Source: CAD feature listing. Evaluate the final solid. Frame: model axes, mm. A direction names the side the tool comes from. Give positions to 0.01 mm unless a question says otherwise; leave off trailing zeros. Write each loop counter-clockwise with the first axis right and the second up, starting at its lowest first coordinate (ties: lowest second). Pieces come first, ordered by that corner, then holes. Notation, with made-up numbers: (-2, 20) -> (30, 20) arc R6 cw to (30, 31) -> close; hole circle Ø11 at (69.5, 66.25). An arc over 180 degrees is marked (long way). Use one line per item in the form item = value. Start each with the question number.
(1) Cut plane B-B, the plane z = -13. Count the separate pieces of the cut face and the enclosed holes in it, and give its area (3 significant figures).
(2) Material intervals for line 1 along Y through (x, z) = (0, 4); line 2 along X through (y, z) = (0, -3); line 3 along Y through (x, z) = (133, -11), sorted ascending. Write a range as from..to.
(3) Set-up query: faces 1 (the face through (100.9, 55.1, 0.3)), 2 (the face through (35.22, 1.93, 0.28)), 3 (the face through (131.72, 80.96, 0.28)). Return all of +Z, -Z, +X, -X, +Y, -Y with unobstructed straight access to the full face (end or side cutting, diameter ignored); none if empty.
(4) First-contact query: P1, Ø1.5, axis at x = 85.5, z = -0.5, coming from the +Y side; P2, Ø12, axis at x = 58, z = -8, coming from the -Y side; P3, Ø4, axis at x = 93, z = -11, coming from the -Y side. Flat tips, straight axial feed; report the tip coordinate or a pass-through.
(5) Draft query along X for faces 4 (the face through (-4.515, -3.462, 0.284)), 5 (the face through (19.249, 26.736, 0.284)), 6 (the face through (125, 83, -20.32)). Return one class per face: pulls with the +X half, pulls with the -X half, needs draft (parallel to the pull), parting line crosses it, or undercut.
(6) Cut plane A-A, the plane x = 0. Output: boundary loops of the cut face in (y, z), and give its area (3 significant figures).
from build123d import *

# Parameters (mm, degrees)
SKETCH1_R                       = 10.16
BOSS_EXTRUDE1_DEPTH             = 20.32
BOSS_EXTRUDE1_DEPTH_BACK        = 20.32
CUT_EXTRUDE2_DEPTH              = 85.09
CUT_EXTRUDE2_DEPTH_BACK         = 85.09
BOSS_EXTRUDE2_REACH             = 22.32
SKETCH4_R                       = 10.16
SKETCH4_R_2                     = 5.690130056
BOSS_EXTRUDE2_DIRECTION_2_REACH = 22.32


with BuildPart() as part:
    # Sketch1 → Boss-Extrude1 (new body, two sides)
    with BuildSketch(Plane.XY) as boss_extrude1_sk:
        with BuildLine():
            Line((-6.540792976, 16.533191684), (60.990787353, 43.249756441))
            Line((60.990787353, 43.249756441), (111.219656073, 79.494763154))
            add(Edge.make_bspline(
                [(111.219656073, 79.494763154), (115.143809103, 89.538582986), (111.485189552, 100.079798905)],
                knots=[0, 0, 0, 1, 1, 1], degree=2))
            add(Edge.make_bspline(
                [(111.485189552, 100.079798905), (118.666753914, 114.310676005), (138.716144692, 104.878983682)],
                knots=[0, 0, 0, 1, 1, 1], degree=2))
            add(Edge.make_bspline(
                [(119.614328761, 100.079798905), (127.464188518, 107.13262314), (138.716144692, 104.878983682)],
                knots=[0, 0, 0, 1, 1, 1], degree=2))
            add(Edge.make_bspline(
                [(124.506668386, 84.517246437), (119.614328761, 100.079798905)],
                knots=[0, 0, 1, 1], degree=1))
            add(Edge.make_bspline(
                [(124.506668386, 84.517246437), (139.137891823, 77.302308665)],
                knots=[0, 0, 1, 1], degree=1))
            add(Edge.make_bspline(
                [(139.137891823, 77.302308665), (147.308308442, 83.981149896), (146.802069804, 95.445404385)],
                knots=[0, 0, 0, 1, 1, 1], degree=2))
            add(Edge.make_bspline(
                [(137.894611709, 69.268806388), (153.056423627, 74.189394673), (146.802069804, 95.445404385)],
                knots=[0, 0, 0, 1, 1, 1], degree=2))
            add(Edge.make_bspline(
                [(117.511141846, 72.154696419), (128.036963673, 74.496569321), (137.894611709, 69.268806388)],
                knots=[0, 0, 0, 1, 1, 1], degree=2))
            Line((117.511141846, 72.154696419), (74.032842511, 27.522572281))
            Line((74.032842511, 27.522572281), (9.788223937, -14.843148998))
            ThreePointArc((9.788223937, -14.843148998), (-15.771973263, -8.208121551), (-6.540792976, 16.533191684))
        make_face()
        Circle(SKETCH1_R, mode=Mode.SUBTRACT)
    extrude(amount=BOSS_EXTRUDE1_DEPTH)
    extrude(boss_extrude1_sk.sketch, amount=-BOSS_EXTRUDE1_DEPTH_BACK)

    # Sketch3 → Cut-Extrude2 (cut, two sides)
    with BuildSketch(Plane(origin=(-6.540792976, 16.533191684, 0), x_dir=(0.929875798, 0.367873621, 0), z_dir=(-0.367873621, 0.929875798, 0))) as cut_extrude2_sk:
        with BuildLine():
            Line((17.521009343, 20.32), (69.311227208, 80.494269298))
            Line((69.311227208, 80.494269298), (134.577572969, 24.523321464))
            add(Edge.make_bspline(
                [(17.521009343, 20.32), (76.642520542, -10.04244022), (134.577572969, 24.523321464)],
                knots=[0, 0, 0, 1, 1, 1], degree=2))
        make_face()
        with BuildLine():
            Line((17.521009343, -20.32), (69.311227208, -80.494269298))
            Line((69.311227208, -80.494269298), (134.577572969, -24.523321464))
            add(Edge.make_bspline(
                [(17.521009343, -20.32), (76.642520542, 10.04244022), (134.577572969, -24.523321464)],
                knots=[0, 0, 0, 1, 1, 1], degree=2))
        make_face()
    extrude(amount=CUT_EXTRUDE2_DEPTH, mode=Mode.SUBTRACT)
    extrude(cut_extrude2_sk.sketch, amount=-CUT_EXTRUDE2_DEPTH_BACK, mode=Mode.SUBTRACT)

    # Boss-Extrude2: up to this face of the body (flat: up to its plane)
    boss_extrude2_end = Plane(part.part.faces().sort_by_distance((-15.269069271, -7.946397985, 20.32))[0])
    # Sketch4 → Boss-Extrude2 (add, up to the picked face)
    with BuildSketch(Plane.XY, mode=Mode.PRIVATE) as boss_extrude2_sk1:
        Circle(SKETCH4_R)
        Circle(SKETCH4_R_2, mode=Mode.SUBTRACT)
    boss_extrude2_tool1 = split(extrude(boss_extrude2_sk1.sketch, amount=BOSS_EXTRUDE2_REACH, mode=Mode.PRIVATE), bisect_by=boss_extrude2_end, keep=Keep.BOTH, mode=Mode.PRIVATE)
    add(boss_extrude2_tool1.solids().sort_by_distance((-9.872632, 0, 0))[0])

    # Boss-Extrude2 direction 2: up to this face of the body (flat: up to its plane)
    boss_extrude2_direction_2_end = Plane(part.part.faces().sort_by_distance((-15.269069271, -7.946397985, -20.32))[0])
    # Sketch4 → Boss-Extrude2 direction 2 (add, up to the picked face)
    with BuildSketch(Plane.XY, mode=Mode.PRIVATE) as boss_extrude2_direction_2_sk1:
        Circle(SKETCH4_R)
        Circle(SKETCH4_R_2, mode=Mode.SUBTRACT)
    boss_extrude2_direction_2_tool1 = split(extrude(boss_extrude2_direction_2_sk1.sketch, amount=-BOSS_EXTRUDE2_DIRECTION_2_REACH, mode=Mode.PRIVATE), bisect_by=boss_extrude2_direction_2_end, keep=Keep.BOTH, mode=Mode.PRIVATE)
    add(boss_extrude2_direction_2_tool1.solids().sort_by_distance((-9.872632, 0, 0))[0])


solid = part.part
Geometry says:
q1.separate_pieces = 2
q1.enclosed_holes = 1
q1.area = 2,420 mm^2
q2.line_1 = -17.78..-5.69, 5.69..19.12
q2.line_2 = -17.78..-5.69, 5.69..32.3
q2.line_3 = 71.38..80.33, 105.42..107.17
q3.face_1 = +Z, -Z, -Y
q3.face_2 = +Z, -Z, +X, -Y
q3.face_3 = +Z, -Z
q4.P1 = 61.48
q4.P2 = 12.99
q4.P3 = 45.17
q5.face_4 = undercut
q5.face_5 = pulls with the -X half
q5.face_6 = needs draft
q6.outline = (-17.78, -20.32) -> (-5.69, -20.32) -> (-5.69, 20.32) -> (-17.78, 20.32) -> close; (5.69, -20.32) -> (19.12, -20.32) -> (19.12, 20.32) -> (5.69, 20.32) -> close
q6.area = 1,040 mm^2
